Autodesk Inventor part; units mm, degrees
ref_plane "YZ Plane" through (0, 0, 0) normal (1, 0, 0) x (0, 1, 0)
ref_plane "XZ Plane" through (0, 0, 0) normal (0, 1, 0) x (-1, 0, 0)
ref_plane "XY Plane" through (0, 0, 0) normal (0, 0, 1) x (1, 0, 0)
sketch "Skizze1" plane through (0, 0, 0) normal (0, 1, 0) x (-1, 0, 0)
  line L0 (0, 0) -> (25, 0)
  line L1 (25, 0) -> (25, 50)
  line L2 (25, 50) -> (0, 50)
  line L3 (0, 42.5) -> (-9.9167, 42.5)
  line L4 (-9.9167, 42.5) -> (-9.9167, 7.5)
  line L5 (-9.9167, 7.5) -> (0, 7.5)
  line L6 (15, 32.5) -> (-5, 32.5)
  line L7 (-5, 32.5) -> (-5, 17.5)
  line L8 (-5, 17.5) -> (15, 17.5)
  line L9 (15, 17.5) -> (15, 32.5)
  line L10 (0, 7.5) -> (0, 17.5)
  line L11 (0, 32.5) -> (0, 42.5)
  line L12 (0, 50) -> (0, 32.5)
  line L13 (0, 17.5) -> (0, 0)
  dimension "d0" = 50
  dimension "d1" = 25
  dimension "d2" = 7.5
  dimension "d4" = 35
  dimension "d5" = 10
  dimension "d6" = 15
  dimension "d8" = 20
  dimension "d9" = 15
extrude "Extrusion1" add sketch "Skizze1" along normal blind 3 contours L13 L10 L8 L9 L6 L11 L12 L2 L1 L0 | L5 L4 L3 L11 L6 L7 L8 L10
sketch "Skizze2" plane through (0, 0, 42.5) normal (0, 0, 1) x (1, 0, 0)
  line L0 (9.9167, 0) -> (9.9167, 3)
  line L1 (9.9167, 3) -> (6.9167, 3)
  line L2 (6.9167, 3) -> (6.9167, 15)
  line L3 (6.9167, 15) -> (9.9167, 15)
  line L4 (9.9167, 15) -> (9.9167, 3)
  point P0 (0, 0)
  dimension "d12" = 3
  dimension "d13" = 12
extrude "Extrusion2" add sketch "Skizze2" against normal up to surface (35 mm away)
fillet "Rundung1" radius 2 1 edges at (6.9167, 3, 25)
sketch "Skizze3" plane through (0, 0, 0) normal (0, -1, 0) x (1, 0, 0)
  line L0 (-22, 0) -> (-7, 0)
  line L1 (-7, 0) -> (-7, 2)
  line L2 (-7, 2) -> (-22, 2)
  line L3 (-22, 2) -> (-22, 0)
  line L4 (-22, 48) -> (-7, 48)
  line L5 (-7, 48) -> (-7, 50)
  line L6 (-7, 50) -> (-22, 50)
  line L7 (-22, 50) -> (-22, 48)
  line L8 (-25, 50) -> (0, 50)
  line L9 (0, 50) -> (0, 42.5)
  point P0 (0, 0)
  dimension "d17" = 2
  dimension "d18" = 2
  dimension "d19" = 46
  dimension "d20" = 15
  dimension "d21" = 15
  dimension "d22" = 0
  dimension "d23" = 7
extrude "Extrusion3" add sketch "Skizze3" along normal blind 6
properties part number "Ultrasonic" material "Stahl, Guss"
CAD build for the part. Positions are in the model's coordinates, mm. A direction names the side the tool comes from. Give positions to 0.01 mm unless a question says otherwise; leave off trailing zeros. Order: outer loops, then holes, each group sorted by start corner. A loop starts at its lowest first (then second) coordinate and runs counter-clockwise, first axis right, second up.
(1) Mould opens along X. For faces 1 (the flat face through (-15, -1, 0)), 2 (the flat face through (-5, 1, 32.5)), 3 (the flat face through (6.917, 10, 25)) say: released by +X, released by -X, zero draft, split by the parting line, or undercut.
(2) Tool access for faces 4 (the flat face through (-7, -3, 49)), 5 (the flat face through (0, 1, 4)), 6 (the flat face through (7.1, 5.9, 42.5)), 7 (the flat face through (5, 1, 25)): list every direction of +Z, -Z, +X, -X, +Y, -Y with a clear straight run to the whole face (end or side of a thin tool).
(3) Saw through at A-A, the plane x = -8. Give the cut face in (y, z).
(4) Saw through at C-C, the plane z = 24.5. Give the cut face in (x, y), then the cut area to 3 significant figures.
(5) Flat gauge pins, fed straight in: pin 1 (1.5 mm diameter, centred on x = -17.5, z = 24, fed in from -Y); pin 2 (2 mm diameter, centred on y = -3, z = 48.5, fed in from -X); pin 3 (8 mm diameter, centred on y = 9.5, z = 16.5, fed in from -X). Where does each tip first touch, or does it go through?
(6) Drill centre lines: L1, parallel to Z at x = -12, y = 1.25; L2, parallel to Z at x = -15.5, y = -2; L3, parallel to Y at x = -20.5, z = 33. Where is each one in solid material? Low to high.
(7) Saw through at B-B, the plane y = -1. Give the cut face in (x, z).
(8) Saw through at D-D, the plane x = -18.5. Give the cut face in (y, z).
Results found:
1. face 1: zero draft
1. face 2: undercut
1. face 3: released by -X
2. face 4: +Z, -Z, +X, -Y
2. face 5: -Z, +X, +Y, -Y
2. face 6: +Z, +X, +Y, -Y
2. face 7: +Y, -Y
3. outline: (-6, 0) - (3, 0) - (3, 17.5) - (0, 17.5) - (0, 2) - (-6, 2) - close; (-6, 48) - (0, 48) - (0, 32.5) - (3, 32.5) - (3, 50) - (-6, 50) - close
4. outline: (-25, 0) - (-15, 0) - (-15, 3) - (-25, 3) - close; (5, 0) - (9.92, 0) - (9.92, 15) - (6.92, 15) - (6.92, 5) arc R2 cw to (5, 3) - close
4. area: 81.6 mm2
5. pin 1: stops at y = 0
5. pin 2: stops at x = -22
5. pin 3: stops at x = 6.92
6. L1: z = 0 to 17.5, 32.5 to 50
6. L2: z = 0 to 2, 48 to 50
6. L3: y = 0 to 3
7. outline: (-22, 0) - (-7, 0) - (-7, 2) - (-22, 2) - close; (-22, 48) - (-7, 48) - (-7, 50) - (-22, 50) - close
8. outline: (-6, 0) - (3, 0) - (3, 50) - (-6, 50) - (-6, 48) - (0, 48) - (0, 2) - (-6, 2) - close
